For this review, take the finished solid that the model builds, in its own axes (mm). Face numbers are marked on the shaded views. Round coordinates to 2 decimals unless told otherwise and drop trailing zeros. Loops run counter-clockwise (first coordinate to the right, second up) from the corner with the lowest first, then second, coordinate; pieces in that order, holes last.
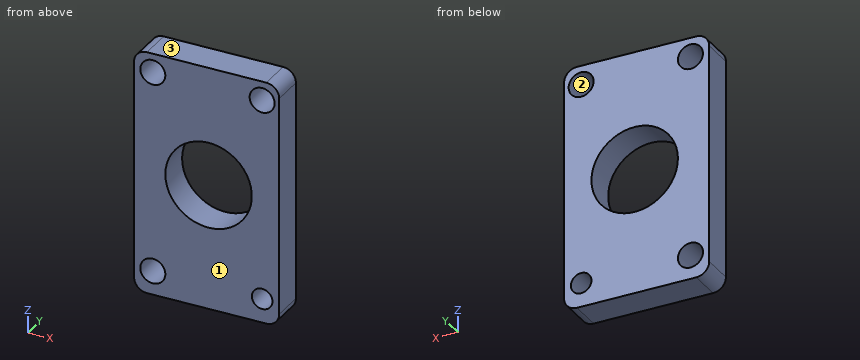
Autodesk Inventor part; units mm, degrees
ref_plane "YZ Plane" through (0, 0, 0) normal (1, 0, 0) x (0, 1, 0)
ref_plane "XZ Plane" through (0, 0, 0) normal (0, 1, 0) x (-1, 0, 0)
ref_plane "XY Plane" through (0, 0, 0) normal (0, 0, 1) x (1, 0, 0)
sketch "Sketch2" plane through (0, 0, 0) normal (0, 1, 0) x (-1, 0, 0)
  line L0 (11.5834, 18.5596) -> (-10.9749, 18.5596)
  line L1 (-10.9749, 18.5596) -> (-10.9749, -19.5593)
  line L2 (-10.9749, -19.5593) -> (11.5834, -19.5593)
  line L3 (11.5834, -19.5593) -> (11.5834, 18.5596)
  circle A0 centre (8.6713, 15.6039) radius 1.9409
  circle A1 centre (0, 0) radius 6.7207
  circle A2 centre (-8.3236, 15.6039) radius 1.9409
  circle A3 centre (8.6713, -15.8213) radius 1.9511
  circle A4 centre (-8.3236, -15.8213) radius 1.6029
extrude "Extrusion2" add sketch "Sketch2" along normal blind 5
fillet "Fillet1" radius 2 1 edges at (-11.5834, 2.5, 18.5596)
fillet "Fillet2" radius 2 1 edges at (10.9749, 2.5, 18.5596)
fillet "Fillet3" radius 2 1 edges at (10.9749, 2.5, -19.5593)
fillet "Fillet4" radius 2 1 edges at (-11.5834, 2.5, -19.5593)
properties part number "Bloque-Part"
(1) The part is to be moulded in two halves that separate along Z. For the marked faces 1, 2 and 3, say which applies: pulls with the +Z half, pulls with the -Z half, needs draft (parallel to the pull), parting line crosses it, or undercut.
(2) Add section B-B (z = 0). Give the boundary of the cut face in (x, y).
(3) For L1, parallel to Z at x = 0, y = 2.15; L2, parallel to Z at x = -8, y = 2.25; L3, parallel to X at y = 1.2, z = -16, list the stretches that pass through material, from the lowest coordinate up.
(4) Insertion check: pin 1 Ø1 at (x, z) = (-8.5, -0.5) entering from -Y; pin 2 Ø1.5 at (x, z) = (-0.5, -5.5) entering from +Y. Each pin has a flat end and moves straight along its axis. Give the tip position at first contact, or say it passes through.
(5) Add section A-A (x = 0). Give the boundary of the cut face in (y, z), plus the area to 3 significant figures.
(6) Add section C-C (y = 2.35). Give the boundary of the cut face in (x, z).
Outcome:
1. face 1: needs draft
1. face 2: undercut
1. face 3: pulls with the +Z half
2. outline: (-11.58, 0) - (-6.72, 0) - (-6.72, 5) - (-11.58, 5) - close; (6.72, 0) - (10.97, 0) - (10.97, 5) - (6.72, 5) - close
3. L1: z = -19.56 to -6.72, 6.72 to 18.56
3. L2: z = -19.56 to -17.65, -13.99 to 13.78, 17.43 to 18.56
3. L3: x = -11.58 to -10.61, -6.73 to 6.73, 9.92 to 10.97
4. pin 1: stops at y = 0
4. pin 2: passes through
5. outline: (0, -19.56) - (5, -19.56) - (5, -6.72) - (0, -6.72) - close; (0, 6.72) - (5, 6.72) - (5, 18.56) - (0, 18.56) - close
5. area: 123 mm2
6. outline: (-11.58, -17.56) arc R2 ccw to (-9.58, -19.56) - (8.97, -19.56) arc R2 ccw to (10.97, -17.56) - (10.97, 16.56) arc R2 ccw to (8.97, 18.56) - (-9.58, 18.56) arc R2 ccw to (-11.58, 16.56) - close; hole circle Ø3.9 at (-8.67, -15.82); hole circle Ø3.88 at (-8.67, 15.6); hole circle Ø13.44 at (0, 0); hole circle Ø3.88 at (8.32, 15.6); hole circle Ø3.21 at (8.32, -15.82)
